The model under review builds one solid part; all positions refer to its coordinate system, in mm. Coordinates: 2 decimals unless noted, no trailing zeros. Order: outer loops, then holes, each group sorted by start corner. A loop starts at its lowest first (then second) coordinate and runs counter-clockwise, first axis right, second up.
```python
from build123d import *

# Parameters (mm, degrees)
SKETCH_R   = 2.127
SKETCH_R_2 = 3.127
PAD_DEPTH  = 1.8542


with BuildPart() as part:
    # Sketch (on Face33 of Binder001) → Pad (new body)
    with BuildSketch(Plane.YZ):
        with BuildLine():
            Line((0, 10), (130.1, 10))
            ThreePointArc((131.3, 8.8), (130.948528, 9.648528), (130.1, 10))
            Line((131.3, 8.8), (131.3, -121.3))
            ThreePointArc((130.1, -122.5), (130.948528, -122.148528), (131.3, -121.3))
            Line((0, -122.5), (130.1, -122.5))
            ThreePointArc((-1.2, -121.3), (-0.848528, -122.148528), (0, -122.5))
            Line((-1.2, 8.8), (-1.2, -121.3))
            ThreePointArc((0, 10), (-0.848528, 9.648528), (-1.2, 8.8))
        make_face()
        with Locations((14.3, 5)):
            Circle(SKETCH_R, mode=Mode.SUBTRACT)
        with Locations((14.3, -117.5)):
            Circle(SKETCH_R, mode=Mode.SUBTRACT)
        with Locations((56.923, -56.25)):
            Circle(SKETCH_R_2, mode=Mode.SUBTRACT)
        with Locations((73.177, -56.25)):
            Circle(SKETCH_R_2, mode=Mode.SUBTRACT)
        with BuildLine():
            Line((31.925, 3.9459), (98.175, 3.9459))
            ThreePointArc((98.175, 3.9459), (99.2291, 5), (98.175, 6.0541))
            Line((98.175, 6.0541), (31.925, 6.0541))
            ThreePointArc((31.925, 6.0541), (30.8709, 5), (31.925, 3.9459))
        make_face(mode=Mode.SUBTRACT)
        with BuildLine():
            ThreePointArc((127.3541, -23.125), (126.3, -22.0709), (125.2459, -23.125))
            Line((125.2459, -23.125), (125.2459, -89.375))
            ThreePointArc((125.2459, -89.375), (126.3, -90.4291), (127.3541, -89.375))
            Line((127.3541, -23.125), (127.3541, -89.375))
        make_face(mode=Mode.SUBTRACT)
        with BuildLine():
            ThreePointArc((31.925, -116.4459), (30.8709, -117.5), (31.925, -118.5541))
            Line((31.925, -118.5541), (98.175, -118.5541))
            ThreePointArc((98.175, -118.5541), (99.2291, -117.5), (98.175, -116.4459))
            Line((31.925, -116.4459), (98.175, -116.4459))
        make_face(mode=Mode.SUBTRACT)
    extrude(amount=-PAD_DEPTH)


solid = part.part
```
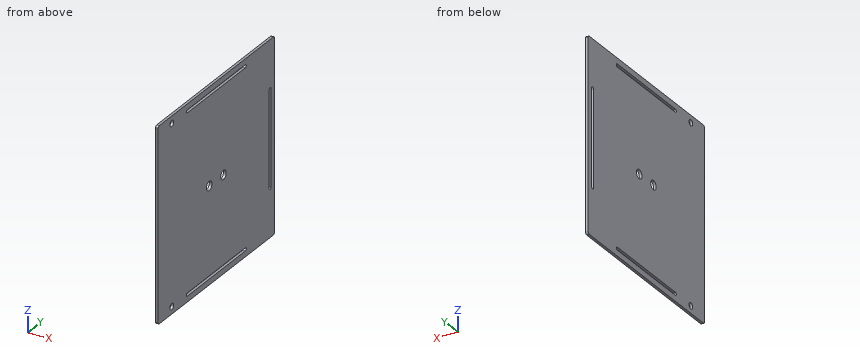
(1) For pin 1 Ø3.5 at (y, z) = (14.3, -117.5) entering from -X, flat-tipped, find the tip position at first contact; note if it passes through.
A:
pin 1: passes through
(2) We need section A-A, the plane y = 14.3. Write out the cut boundary in (x, z), and give its area (3 significant figures).
A:
outline: (-1.85, -122.5) - (0, -122.5) - (0, -119.63) - (-1.85, -119.63) - close; (-1.85, -115.37) - (0, -115.37) - (0, 2.87) - (-1.85, 2.87) - close; (-1.85, 7.13) - (0, 7.13) - (0, 10) - (-1.85, 10) - close
area: 230 mm2
(3) We need section D-D, the plane y = 56. Write out the cut boundary in (x, z), and give its area (3 significant figures).
A:
outline: (-1.85, -122.5) - (0, -122.5) - (0, -118.55) - (-1.85, -118.55) - close; (-1.85, -116.45) - (0, -116.45) - (0, -59.24) - (-1.85, -59.24) - close; (-1.85, -53.26) - (0, -53.26) - (0, 3.95) - (-1.85, 3.95) - close; (-1.85, 6.05) - (0, 6.05) - (0, 10) - (-1.85, 10) - close
area: 227 mm2
(4) We need section B-B, the plane z = -87. Write out the cut boundary in (x, y).
A:
outline: (-1.85, -1.2) - (0, -1.2) - (0, 125.25) - (-1.85, 125.25) - close; (-1.85, 127.35) - (0, 127.35) - (0, 131.3) - (-1.85, 131.3) - close
(5) We need section C-C, the plane z = -56.25. Write out the cut boundary in (x, y).
A:
outline: (-1.85, -1.2) - (0, -1.2) - (0, 53.8) - (-1.85, 53.8) - close; (-1.85, 60.05) - (0, 60.05) - (0, 70.05) - (-1.85, 70.05) - close; (-1.85, 76.3) - (0, 76.3) - (0, 125.25) - (-1.85, 125.25) - close; (-1.85, 127.35) - (0, 127.35) - (0, 131.3) - (-1.85, 131.3) - close
(6) Wall thickness on probe 1 along Z at (x, y) = (-1.35, 41); probe 2 along Z at (x, y) = (-1.3, 14.3); probe 3 along Z at (x, y) = (-0.4, 56): over which ranges is each line inside the solid? List them lowest first.
A:
probe 1: z = -122.5 to -118.55, -116.45 to 3.95, 6.05 to 10
probe 2: z = -122.5 to -119.63, -115.37 to 2.87, 7.13 to 10
probe 3: z = -122.5 to -118.55, -116.45 to -59.24, -53.26 to 3.95, 6.05 to 10
